from build123d import *

# Parameters (mm, degrees)
F0_R     = 5.08
F1_DEPTH = 6.35


with BuildPart() as f1:
    # F0 (on Front) → F1 (new body)
    with BuildSketch(Plane.XZ):
        Polygon((192.247183, -65.812313), (0, 0), (-192.247183, -65.812313), (-216.278081, -74.038852), (-207.854538, -98.645227), (0, -25.4), (207.854538, -98.645227), (216.278081, -74.038852), align=None)
        with BuildLine():
            Line((-216.278081, -74.038852), (-192.247183, -65.812313))
            ThreePointArc((-192.247183, -65.812313), (-168.935929, 112.919847), (-12.7, 202.802737))
            Line((-12.7, 202.802737), (-12.7, 228.24695))
            ThreePointArc((-12.7, 228.24695), (-189.609907, 127.695118), (-216.278081, -74.038852))
        make_face()
        with Locations((-101.6, 190.14695)):
            Circle(F0_R, mode=Mode.SUBTRACT)
        with BuildLine():
            ThreePointArc((12.7, 202.802737), (168.935929, 112.919847), (192.247183, -65.812313))
            Line((192.247183, -65.812313), (216.278081, -74.038852))
            ThreePointArc((216.278081, -74.038852), (189.609907, 127.695118), (12.7, 228.24695))
            Line((12.7, 228.24695), (12.7, 202.802737))
        make_face()
        with Locations((101.6, 190.14695)):
            Circle(F0_R, mode=Mode.SUBTRACT)
        with BuildLine():
            Line((-12.7, 228.24695), (-12.7, 202.802737))
            ThreePointArc((-12.7, 202.802737), (0, 203.2), (12.7, 202.802737))
            Line((12.7, 202.802737), (12.7, 228.24695))
            ThreePointArc((12.7, 228.24695), (0, 228.6), (-12.7, 228.24695))
        make_face()
        with BuildLine():
            ThreePointArc((12.7, 202.802737), (0, 203.2), (-12.7, 202.802737))
            Line((-12.7, 202.802737), (-12.7, 139.34695))
            Line((-12.7, 139.34695), (12.7, 139.34695))
            Line((12.7, 139.34695), (12.7, 202.802737))
        make_face()
    extrude(amount=F1_DEPTH)


solid = f1.part
Could you check a few things on this model? Use its own coordinates, in mm. A direction names the side the tool comes from. Give positions to 0.01 mm unless a question says otherwise; leave off trailing zeros. Loops run counter-clockwise (first coordinate to the right, second up) from the corner with the lowest first, then second, coordinate; pieces in that order, holes last. Notation, with made-up numbers: M 55.5,44.5 L 105.5,44.5 A22 ccw 105.5,77.5 Z; hole C 31.25,-21 d7. An arc over 180 degrees is marked long. Answer as a JSON object with one key per item and string values.
Q1. For P1, Ø3, axis at y = -2, z = 181.5, coming from the -X side; P2, Ø1.9, axis at y = -1.5, z = 159, coming from the +X side; P3, Ø1, axis at y = -3, z = 120.5, coming from the -X side, each with a flat end and sliding along its axis, tell me the tip position at first contact or that it passes through.
Values found:
{"P1": "stops at x = -140.92", "P2": "stops at x = 165.16", "P3": "stops at x = -194.57"}
Q2. For faces 1 (the flat face through (102.47, -3.13, -61.51)), 2 (the cylindrical face through (191.24, -3.13, 125.24)), 3 (the flat face through (97.469, -3.131, -33.367)), which set-ups out of +Z, -Z, +X, -X, +Y, -Y let a thin tool reach every point of the face, with its end or its side?
Values found:
{"face 1": "-Z, +Y, -Y", "face 2": "+X, +Y, -Y", "face 3": "+Y, -Y"}
Q3. Suppose I cut it at A-A, the plane x = -101.6. List the corners of the cut face in (y, z) for me, plus the area to 3 significant figures.
Values found:
{"outline": "M -6.35,-61.2 L 0,-61.2 L 0,-34.78 L -6.35,-34.78 Z; M -6.35,175.98 L 0,175.98 L 0,185.07 L -6.35,185.07 Z; M -6.35,195.23 L 0,195.23 L 0,204.78 L -6.35,204.78 Z", "area": "286 mm²"}
Q4. Suppose I cut it at B-B, the plane z = -49.5. List the corners of the cut face in (x, y) for me.
Values found:
{"outline": "M -223.18,-6.35 L -197.08,-6.35 L -197.08,0 L -223.18,0 Z; M -144.6,-6.35 L -68.39,-6.35 L -68.39,0 L -144.6,0 Z; M 68.39,-6.35 L 144.6,-6.35 L 144.6,0 L 68.39,0 Z; M 197.08,-6.35 L 223.18,-6.35 L 223.18,0 L 197.08,0 Z"}
Q5. If we mould it in two halves opening along Z, with no side actions, what happens to faces 4 (the cylindrical face through (-170.4, -3.1, 110.7)), 5 (the flat face through (-94.778, -3.131, -32.445)), 6 (the flat face through (-105.382, -3.131, -62.535)), 7 (the flat face through (-18, 0, -7))? For each: pulls with the +Z half, pulls with the -Z half, needs draft (parallel to the pull), parting line crosses it, or undercut.
Values found:
{"face 4": "undercut", "face 5": "undercut", "face 6": "pulls with the -Z half", "face 7": "needs draft"}
Q6. Suppose I cut it at C-C, the plane x = -33. List the corners of the cut face in (y, z) for me.
Values found:
{"outline": "M -6.35,-37.03 L 0,-37.03 L 0,-11.3 L -6.35,-11.3 Z; M -6.35,200.5 L 0,200.5 L 0,226.21 L -6.35,226.21 Z"}
Q7. If I drill on probe 1 along X at (y, z) = (-0.75, 173); probe 2 along X at (y, z) = (-6, 180); probe 3 along Z at (x, y) = (101.6, -4.75), over which ranges is the centre line in solid material (lowest first)? Write a range as [from, to].
Values found:
{"probe 1": "x = [-149.43, -106.59], [-12.7, 12.7], [106.59, 149.43]", "probe 2": "x = [-140.92, -94.29], [-12.7, 12.7], [94.29, 140.92]", "probe 3": "z = [-61.2, -34.78], [175.98, 185.07], [195.23, 204.78]"}
Q8. Suppose I cut it at D-D, the plane z = 11.5. List the corners of the cut face in (x, y) for me.
Values found:
{"outline": "M -228.31,-6.35 L -202.87,-6.35 L -202.87,0 L -228.31,0 Z; M 202.87,-6.35 L 228.31,-6.35 L 228.31,0 L 202.87,0 Z"}
